Answer from the drawing. Dimensions are ordinates in mm from the lowest x, y and z of the part. A direction names the side the tool comes from. Coordinates: 2 decimals unless noted, no trailing zeros. Write each loop counter-clockwise with the first axis right and the second up, starting at its lowest first coordinate (ties: lowest second). Pieces come first, ordered by that corner, then holes.
1) The part is cut by section B-B (y = 21). Determine the outline of the cut face in (x, z), then the cut area to 3 significant figures.
2) Determine the mould class of the marked faces 1, 2, 3 and 4 for opening direction Y: +Y half, -Y half, draft (parallel to the pull), parting line (faces both ways), or undercut.
3) Which of the six approach directions +Z, -Z, +X, -X, +Y, -Y give full straight-line access (tool end or side, diameter ignored) to the marked faces 5, 6 and 7?
4) Find the intervals of material crossed by line 1 (Y direction, x = 14, z = 17.25); line 2 (Y direction, x = 31, z = 16.25); line 3 (X direction, y = 3.5, z = 10), in increasing order.
5) The part is cut by section A-A (z = 14.75). Determine the outline of the cut face in (x, y).
6) The part is cut by section C-C (x = 25). Determine the outline of the cut face in (y, z), then the cut area to 3 significant figures.
7) Each of these flat-tipped pins is pushed along its axis until it touches: pin 1 Ø5.5 at (x, z) = (26.5, 11) entering from -Y; pin 2 Ø2 at (x, y) = (6.5, 8) entering from -Z; pin 3 Ø5.5 at (y, z) = (13.5, 6) entering from +X. Where does it stop, or does it pass through?
8) The part is cut by section D-D (y = 27.5). Determine the outline of the cut face in (x, z).
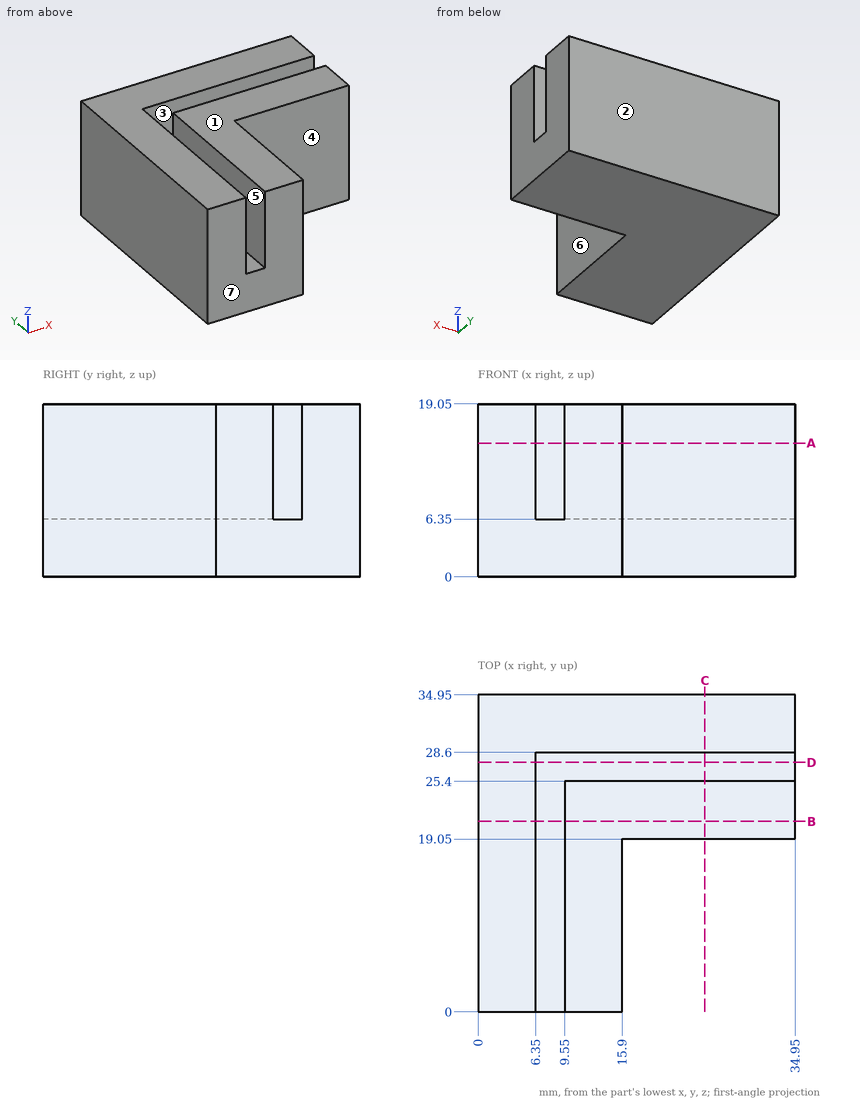
Reported:
1. outline: (0, 0) - (34.95, 0) - (34.95, 19.05) - (9.55, 19.05) - (9.55, 6.35) - (6.35, 6.35) - (6.35, 19.05) - (0, 19.05) - close
1. area: 625 mm2
2. face 1: draft
2. face 2: +Y half
2. face 3: undercut
2. face 4: -Y half
3. face 5: +Z, -Y
3. face 6: +Z, -Z, +X, -Y
3. face 7: +Z, -Z, +X, -X, -Y
4. line 1: y = 0 to 25.4, 28.6 to 34.95
4. line 2: y = 19.05 to 25.4, 28.6 to 34.95
4. line 3: x = 0 to 6.35, 9.55 to 15.9
5. outline: (0, 0) - (6.35, 0) - (6.35, 28.6) - (34.95, 28.6) - (34.95, 34.95) - (0, 34.95) - close; (9.55, 0) - (15.9, 0) - (15.9, 19.05) - (34.95, 19.05) - (34.95, 25.4) - (9.55, 25.4) - close
6. outline: (19.05, 0) - (34.95, 0) - (34.95, 19.05) - (28.6, 19.05) - (28.6, 6.35) - (25.4, 6.35) - (25.4, 19.05) - (19.05, 19.05) - close
6. area: 262 mm2
7. pin 1: stops at y = 19.05
7. pin 2: stops at z = 0
7. pin 3: stops at x = 15.9
8. outline: (0, 0) - (34.95, 0) - (34.95, 6.35) - (6.35, 6.35) - (6.35, 19.05) - (0, 19.05) - close
